Verification items for the finished model (mm, model axes). Face numbers are marked on the shaded views. Give positions to 0.01 mm unless a question says otherwise; leave off trailing zeros. Loops run counter-clockwise (first coordinate to the right, second up) from the corner with the lowest first, then second, coordinate; pieces in that order, holes last. Notation, with made-up numbers: M 51,3 L 100,3 A31 cw 100,27 Z; hole C 24,27 d10. An arc over 180 degrees is marked long. Use a Markdown table: item, result.
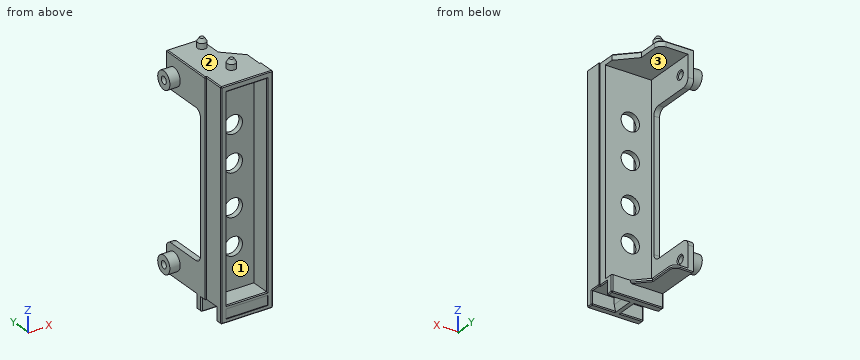
from build123d import *

# Parameters (mm, degrees)
PAD_DEPTH          = 97.8
PAD001_DEPTH       = 2.5
SKETCH002_W        = 22.6
SKETCH002_H        = 4.2
PAD002_DEPTH       = 7.2
PAD003_DEPTH       = 1.2
PAD004_DEPTH       = 2.5
SKETCH005_W        = 10.4
SKETCH005_H        = 8.8
SKETCH005_W_2      = 9.8
POCKET_DEPTH       = 5.8
CHAMFER_SIZE2      = 3
CHAMFER_SIZE       = 0.6
CHAMFER001_SIZE2   = 3
CHAMFER001_SIZE    = 0.6
SKETCH006_R        = 3.9
PAD005_DEPTH       = 4.5
SKETCH007_R        = 1.6
POCKET001_DEPTH    = 5
SKETCH008_R        = 1.9
PAD006_DEPTH       = 4
CHAMFER002_1_SIZE2 = 1
CHAMFER002_1_SIZE  = 1.6
CHAMFER002_2_SIZE2 = 1
CHAMFER002_2_SIZE  = 1.6
SKETCH009_W        = 18.4
SKETCH009_H        = 4.2
POCKET002_DEPTH    = 0.4
SKETCH010_W        = 17.6
SKETCH010_H        = 87.9
POCKET003_DEPTH    = 8.5
CHAMFER003_SIZE    = 0.4
CHAMFER004_SIZE    = 0.4
CHAMFER005_SIZE    = 0.4
SKETCH011_R        = 4
POCKET004_DEPTH    = 5


with BuildPart() as part:
    # Sketch → Pad (new body)
    with BuildSketch(Plane.XY):
        Polygon((-22.6, 0), (-22.6, 9.5), (-23.2, 9.5), (-23.2, 10.8), (-0.6, 10.8), (-0.6, 7.5), (0, 7.5), (0, 0), align=None)
    extrude(amount=PAD_DEPTH)

    # Sketch001 (on Face10 of Pad) → Pad001 (join)
    with BuildSketch(Plane.XY.offset(97.8)):
        with BuildLine():
            Line((-23.2, 10.8), (-23.2, 34.3))
            Line((-23.2, 34.3), (-11.2, 34.3))
            ThreePointArc((-8.2, 31.3), (-9.07868, 33.42132), (-11.2, 34.3))
            Line((-8.2, 31.3), (-8.2, 22.7))
            Line((-8.2, 22.7), (-0.6, 15.1))
            Line((-0.6, 15.1), (-0.6, 10.8))
            Line((-0.6, 10.8), (-23.2, 10.8))
        make_face()
    extrude(amount=-PAD001_DEPTH)

    # Sketch002 (on Face4 of Pad001) → Pad002 (join)
    with BuildSketch(Plane(origin=(0, 0, 0), x_dir=(1, 0, 0), z_dir=(0, 0, -1))):
        with Locations((-11.9, -12.9)):
            Rectangle(SKETCH002_W, SKETCH002_H)
    extrude(amount=-PAD002_DEPTH)

    # Sketch003 (on Face22 of Pad002) → Pad003 (join)
    with BuildSketch(Plane.XY.offset(7.2)):
        with BuildLine():
            Line((-23.2, 15), (-23.2, 34.3))
            Line((-23.2, 34.3), (-17.4, 34.3))
            ThreePointArc((-14.4, 31.3), (-15.27868, 33.42132), (-17.4, 34.3))
            Line((-14.4, 31.3), (-14.4, 20.7))
            Line((-14.4, 20.7), (-8.7, 15))
            Line((-8.7, 15), (-23.2, 15))
        make_face()
    extrude(amount=-PAD003_DEPTH)

    # Sketch004 (on Face7 of Pad003) → Pad004 (join)
    with BuildSketch(Plane(origin=(-23.2, 0, 0), x_dir=(0, -1, 0), z_dir=(-1, 0, 0))):
        with BuildLine():
            Line((-34.3, 7.2), (-34.3, 16.7))
            ThreePointArc((-31.3, 19.7), (-33.42132, 18.82132), (-34.3, 16.7))
            Line((-31.3, 19.7), (-15.4, 19.7))
            ThreePointArc((-15.4, 19.7), (-13.27868, 20.57868), (-12.4, 22.7))
            Line((-12.4, 22.7), (-12.4, 79.8))
            ThreePointArc((-12.4, 79.8), (-13.27868, 81.92132), (-15.4, 82.8))
            Line((-15.4, 82.8), (-31.3, 82.8))
            ThreePointArc((-34.3, 85.8), (-33.42132, 83.67868), (-31.3, 82.8))
            Line((-34.3, 85.8), (-34.3, 95.3))
            Line((-34.3, 95.3), (-10.8, 95.3))
            Line((-10.8, 95.3), (-10.8, 7.2))
            Line((-10.8, 7.2), (-34.3, 7.2))
        make_face()
    extrude(amount=-PAD004_DEPTH)

    # Sketch005 (on Face4 of Pad004) → Pocket (cut)
    with BuildSketch(Plane(origin=(0, 0, 0), x_dir=(1, 0, 0), z_dir=(0, 0, -1))):
        with Locations((-18, -7.4)):
            Rectangle(SKETCH005_W, SKETCH005_H)
        with Locations((-4.9, -7.4)):
            Rectangle(SKETCH005_W_2, SKETCH005_H)
    extrude(amount=-POCKET_DEPTH, mode=Mode.SUBTRACT)

    # Chamfer
    chamfer_edges = [part.edges().sort_by_distance(p)[0] for p in [
        (-9.8, 6.9, 0),
    ]]
    chamfer_side = part.faces().sort_by_distance((-11.3, 2.885526, 0))[0]
    chamfer(chamfer_edges, length=CHAMFER_SIZE, length2=CHAMFER_SIZE2, reference=chamfer_side)

    # Chamfer001
    chamfer001_edges = [part.edges().sort_by_distance(p)[0] for p in [
        (-12.8, 6.9, 0),
    ]]
    chamfer001_side = part.faces().sort_by_distance((-11.36491, 2.668377, 0))[0]
    chamfer(chamfer001_edges, length=CHAMFER001_SIZE, length2=CHAMFER001_SIZE2, reference=chamfer001_side)

    # Sketch006 (on Face25 of Chamfer001) → Pad005 (join)
    with BuildSketch(Plane(origin=(-23.2, 0, 0), x_dir=(0, -1, 0), z_dir=(-1, 0, 0))):
        with Locations((-29.3, 89)):
            Circle(SKETCH006_R)
        with Locations((-29.3, 13)):
            Circle(SKETCH006_R)
    extrude(amount=PAD005_DEPTH)

    # Sketch007 (on Face25 of Pad005) → Pocket001 (cut, symmetric)
    with BuildSketch(Plane(origin=(-23.2, 0, 0), x_dir=(0, -1, 0), z_dir=(-1, 0, 0))):
        with Locations((-29.3, 13)):
            Circle(SKETCH007_R)
        with Locations((-29.3, 89)):
            Circle(SKETCH007_R)
    extrude(amount=POCKET001_DEPTH, both=True, mode=Mode.SUBTRACT)

    # Sketch008 (on Face22 of Pocket001) → Pad006 (join)
    with BuildSketch(Plane.XY.offset(97.8)):
        with Locations((-11.3, 10)):
            Circle(SKETCH008_R)
        with Locations((-11.3, 29)):
            Circle(SKETCH008_R)
    extrude(amount=PAD006_DEPTH)

    # Chamfer002 1
    chamfer002_1_edges = [part.edges().sort_by_distance(p)[0] for p in [
        (-13.2, 29, 101.8),
    ]]
    chamfer002_1_side = part.faces().sort_by_distance((-13.2, 29, 99.8))[0]
    chamfer(chamfer002_1_edges, length=CHAMFER002_1_SIZE, length2=CHAMFER002_1_SIZE2, reference=chamfer002_1_side)

    # Chamfer002 2
    chamfer002_2_edges = [part.edges().sort_by_distance(p)[0] for p in [
        (-13.2, 10, 101.8),
    ]]
    chamfer002_2_side = part.faces().sort_by_distance((-13.2, 10, 99.8))[0]
    chamfer(chamfer002_2_edges, length=CHAMFER002_2_SIZE, length2=CHAMFER002_2_SIZE2, reference=chamfer002_2_side)

    # Sketch009 (on Face12 of Chamfer002) → Pocket002 (cut)
    with BuildSketch(Plane.XZ):
        with Locations((-11.3, 3.7)):
            Rectangle(SKETCH009_W, SKETCH009_H)
    extrude(amount=-POCKET002_DEPTH, mode=Mode.SUBTRACT)

    # Sketch010 (on Face12 of Pocket002) → Pocket003 (cut)
    with BuildSketch(Plane.XZ):
        with Locations((-11.3, 51.15)):
            Rectangle(SKETCH010_W, SKETCH010_H)
    extrude(amount=-POCKET003_DEPTH, mode=Mode.SUBTRACT)

    # Chamfer003
    chamfer003_edges = [part.edges().sort_by_distance(p)[0] for p in [
        (-20.7, 30.9, 13),
        (-20.7, 30.9, 89),
    ]]
    chamfer(chamfer003_edges, length=CHAMFER003_SIZE)

    # Chamfer004
    chamfer004_edges = [part.edges().sort_by_distance(p)[0] for p in [
        (-22.6, 0, 48.9),
        (0, 0, 48.9),
        (-20.1, 0, 51.15),
        (-11.3, 0, 95.1),
        (-2.5, 0, 51.15),
        (-11.3, 0, 7.2),
        (-11.3, 0, 0),
        (0, 1.5, 0),
        (-22.6, 1.5, 0),
        (-17.7, 3, 0),
        (-4.9, 3, 0),
        (-5.2, 11.8, 0),
        (-0.6, 13.4, 0),
        (-0.6, 15, 3.6),
        (-11.9, 15, 0),
        (-18, 11.8, 0),
        (-23.2, 13.4, 0),
        (-23.2, 15, 3),
        (-11.3, 0, 97.8),
        (-22.6, 4.75, 97.8),
        (-22.9, 9.5, 97.8),
        (-23.2, 10.15, 97.8),
        (-23.2, 22.55, 97.8),
        (0, 3.75, 97.8),
        (-0.3, 7.5, 97.8),
        (-0.6, 9.15, 97.8),
        (-0.6, 12.95, 97.8),
        (-4.4, 18.9, 97.8),
        (-8.2, 27, 97.8),
        (0, 3, 2.9),
        (0, 5.25, 5.8),
        (-0.3, 7.5, 5.8),
        (-0.6, 9.15, 5.8),
        (-0.6, 11.3, 5.8),
        (-0.6, 11.8, 2.9),
        (-22.6, 3, 2.9),
        (-22.6, 6.25, 5.8),
        (-22.9, 9.5, 5.8),
        (-23.2, 10.15, 5.8),
        (-23.2, 11.3, 5.8),
        (-23.2, 11.8, 2.9),
    ]]
    chamfer(chamfer004_edges, length=CHAMFER004_SIZE)

    # Chamfer005
    chamfer005_edges = [part.edges().sort_by_distance(p)[0] for p in [
        (-11.55, 17.85, 6),
        (-14.4, 26, 6),
        (-15.27868, 33.42132, 6),
        (-20.3, 34.3, 6),
        (-23.2, 24.65, 6),
    ]]
    chamfer(chamfer005_edges, length=CHAMFER005_SIZE)

    # Sketch011 (on Face22 of Chamfer005) → Pocket004 (cut)
    with BuildSketch(Plane(origin=(0, 10.8, 0), x_dir=(-1, 0, 0), z_dir=(0, 1, 0))):
        with Locations((11.5, 25)):
            Circle(SKETCH011_R)
        with Locations((11.5, 40.9)):
            Circle(SKETCH011_R)
        with Locations((11.5, 59.3)):
            Circle(SKETCH011_R)
        with Locations((11.5, 75.2)):
            Circle(SKETCH011_R)
    extrude(amount=-POCKET004_DEPTH, mode=Mode.SUBTRACT)


solid = part.part
(1) Cross-section at A-A on z = 13. Record the cut outline in (x, y), then the cut area to 3 significant figures.
Results below:
| item | result |
|---|---|
| outline | M -27.7,25.4 L -23.2,25.4 L -23.2,9.5 L -22.6,9.5 L -22.6,0.4 L -22.2,0 L -20.5,0 L -20.1,0.4 L -20.1,8.5 L -2.5,8.5 L -2.5,0.4 L -2.1,0 L -0.4,0 L 0,0.4 L 0,7.5 L -0.6,7.5 L -0.6,10.8 L -20.7,10.8 L -20.7,27.3 L -21.1,27.7 L -27.7,27.7 Z; M -27.7,30.9 L -21.1,30.9 L -20.7,31.3 L -20.7,34.3 L -23.2,34.3 L -23.2,33.2 L -27.7,33.2 Z |
| area | 164 mm^2 |
(2) Draft check along Z on the marked faces 1, 2 and 3. Enter one of: +Z half, -Z half, draft (parallel to the pull), parting line (faces both ways), or undercut.
Results below:
| item | result |
|---|---|
| face 1 | undercut |
| face 2 | +Z half |
| face 3 | undercut |
(3) Gauge pin test, flat ends, axial feed: P1, Ø8, axis at x = -18.5, y = 22.5, coming from the +Z side; P2, Ø1.5, axis at y = 14.5, z = 22.5, coming from the +X side; P3, Ø10.5, axis at x = -11.5, z = 75.2, coming from the -Y side; P4, Ø2.5, axis at y = 4, z = 54, coming from the -X side. Record the tip position at first contact, or that the pin passes through.
Results below:
| item | result |
|---|---|
| P1 | z = 97.8 |
| P2 | through |
| P3 | y = 8.5 |
| P4 | x = -22.6 |
(4) Cross-section at D-D on z = 84. Record the cut outline in (x, y), then the cut area to 3 significant figures.
Results below:
| item | result |
|---|---|
| outline | M -23.2,9.5 L -22.6,9.5 L -22.6,0.4 L -22.2,0 L -20.5,0 L -20.1,0.4 L -20.1,8.5 L -2.5,8.5 L -2.5,0.4 L -2.1,0 L -0.4,0 L 0,0.4 L 0,7.5 L -0.6,7.5 L -0.6,10.8 L -20.7,10.8 L -20.7,33.7 L -23.2,33.7 Z |
| area | 150 mm^2 |
(5) Material ranges on line 1 (Z direction, x = -11.5, y = 10.1); line 2 (Z direction, x = -22.75, y = 29.3); line 3 (X direction, y = 8, z = 92.5), recorded low to high.
Results below:
| item | result |
|---|---|
| line 1 | 0 to 21, 29 to 36.9, 44.9 to 55.3, 63.3 to 71.2, 79.2 to 101.8 |
| line 2 | 6 to 11.4, 14.6 to 19.7, 82.8 to 87.4, 90.6 to 97.8 |
| line 3 | -22.6 to -20.1, -2.5 to -0.6 |
(6) Cross-section at C-C on y = 13.5. Record the cut outline in (x, z).
Results below:
| item | result |
|---|---|
| outline | M -23.2,0.4 L -22.8,0 L -1,0 L -0.6,0.4 L -0.6,7.2 L -20.7,7.2 L -20.7,20.38 L -23.2,20.38 Z; M -23.2,82.12 L -20.7,82.12 L -20.7,95.3 L -0.6,95.3 L -0.6,97.4 L -1,97.8 L -22.8,97.8 L -23.2,97.4 Z |
(7) Cross-section at B-B on x = -25.75. Record the cut outline in (y, z).
Results below:
| item | result |
|---|---|
| outline | C 29.3,13 d7.8; C 29.3,89 d7.8; hole C 29.3,13 d3.2; hole C 29.3,89 d3.2 |
